The figure shows three views and two pictorial views of one solid part (mm, origin at its lowest corner). Answer the questions. A direction names the side the tool comes from. Round coordinates to 2 decimals unless told otherwise and drop trailing zeros. Order: outer loops, then holes, each group sorted by start corner. A loop starts at its lowest first (then second) coordinate and runs counter-clockwise, first axis right, second up. Notation, with made-up numbers: (-21.75, 63) - (27.25, 63) arc R21 ccw to (27.25, 81) - close; hole circle Ø1 at (29.5, 56.25). An arc over 180 degrees is marked (long way). Write item = value, one per line.
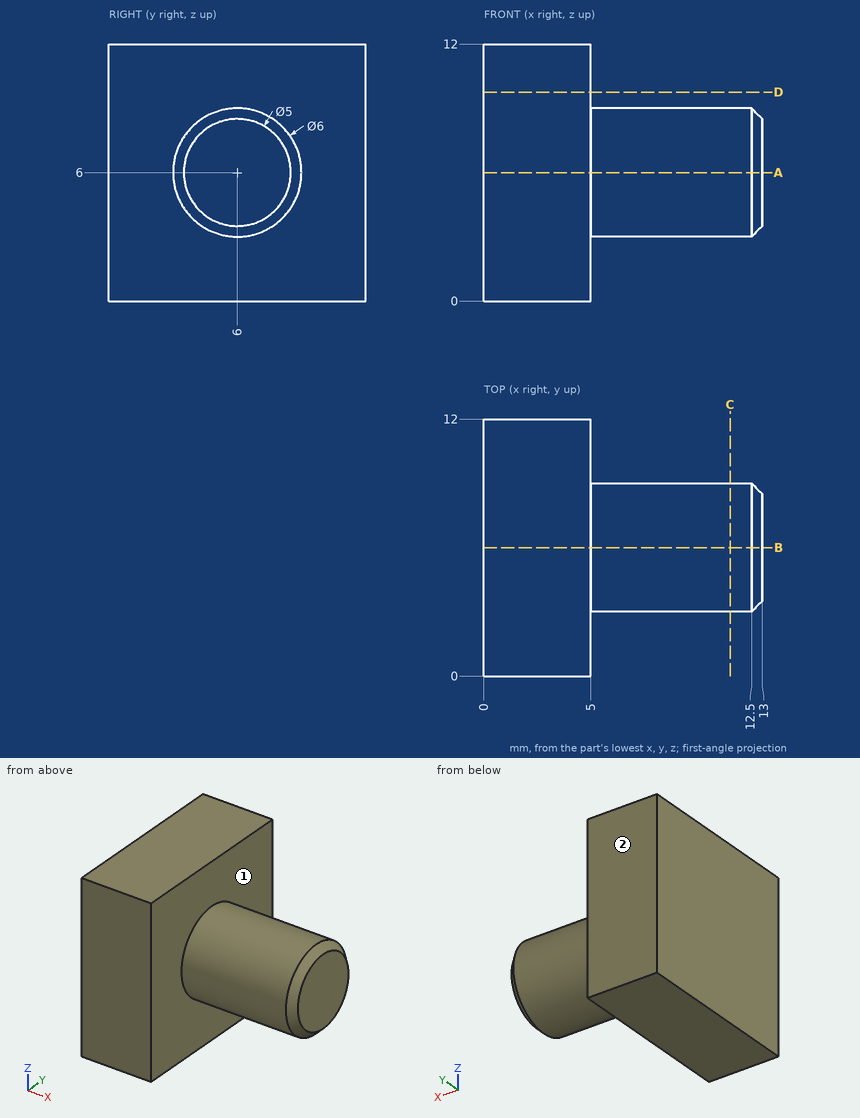
Q1. Section C-C on x = 11.5 is taken. Determine the outline of the cut face in (y, z).
Model answer:
outline = circle Ø6 at (6, 6)
Q2. Flat-ended cylindrical pins translate along their axes: P1, Ø1.5, axis at x = 5, z = 9.5, coming from the -Y side; P2, Ø1, axis at x = 9.5, z = 3.5, coming from the +Y side; P3, Ø2, axis at x = 6.5, z = 8.5, coming from the -Y side. Find the tip coordinate at first contact, or state that the pin passes through.
Model answer:
P1 = 0
P2 = 8.24
P3 = 3.4
Q3. For the marked faces 1 and 2, determine the directions among +Z, -Z, +X, -X, +Y, -Y from which every point of the face is accessible in a straight line to the end or side of a thin tool.
Model answer:
face_1 = +X
face_2 = +Z, -Z, +X, -X, +Y
Q4. Section A-A on z = 6 is taken. Determine the outline of the cut face in (x, y).
Model answer:
outline = (0, 0) - (5, 0) - (5, 3) - (12.5, 3) - (13, 3.5) - (13, 8.5) - (12.5, 9) - (5, 9) - (5, 12) - (0, 12) - close
Q5. Section D-D on z = 9.75 is taken. Determine the outline of the cut face in (x, y), then the cut area to 3 significant figures.
Model answer:
outline = (0, 0) - (5, 0) - (5, 12) - (0, 12) - close
area = 60.0 mm^2
Q6. Find the intervals of material crossed by line 1 (X direction, y = 7.75, z = 3); line 2 (Z direction, x = 9.5, y = 5.75); line 3 (Z direction, x = 6.75, y = 5), in increasing order. Write a range as from..to.
Model answer:
line_1 = 0..5
line_2 = 3.01..8.99
line_3 = 3.17..8.83
